Here's how the part is built. I have some questions about the finished solid (model axes, mm). Round coordinates to 2 decimals unless told otherwise and drop trailing zeros. Order: outer loops, then holes, each group sorted by start corner. A loop starts at its lowest first (then second) coordinate and runs counter-clockwise, first axis right, second up. Notation, with made-up numbers: (47, -4.75) -> (81, -4.75) arc R36 ccw to (81, 31.25) -> close; hole circle Ø8 at (87.25, 3). An arc over 180 degrees is marked (long way). Use a Markdown table: item, result. Add a question column.
(1) I want a section at D-D, the plane y = -31.5. Please give me the cut outline in (x, z).
(2) I want a section at C-C, the plane x = 13.5. Please give me the cut outline in (y, z).
(3) I want a section at B-B, the plane z = 0. Please give me the cut outline in (x, y).
(4) I want a section at A-A, the plane y = 66. Please give me the cut outline in (x, z).
(5) If I drill on probe 1 along X at (y, z) = (63.5, -5); probe 2 along Y at (x, z) = (1209, -74.5); probe 3 along X at (y, z) = (-22.5, 3.5), over which ranges is the centre line in solid material (lowest first)?
(6) I'm going to push flat-ended pins straight in: P1, Ø8, axis at y = 6, z = 33.5, coming from the +X side; P2, Ø5, axis at y = 93, z = -44.5, coming from the -X side; P3, Ø3, axis at y = -29.5, z = -15.5, coming from the +X side. Where does each tip first touch, or does it pass through?
from build123d import *

# Parameters (mm, degrees)
BOSS_EXTRUDE1_DEPTH = 100
SKETCH3_R           = 50
BOSS_EXTRUDE3_DEPTH = 50
SKETCH2_W           = 100
SKETCH2_H           = 100
CUT_EXTRUDE1_DEPTH  = 100
SKETCH4_W           = 200
SKETCH4_H           = 200
CUT_EXTRUDE2_DEPTH  = 10


with BuildPart() as part:
    # Sketch1 → Boss-Extrude1 (new body)
    with BuildSketch(Plane(origin=(0, 0, 0), x_dir=(1, 0, 0), z_dir=(0, 1, 0))):
        with BuildLine():
            Line((0, 150), (1150, 150))
            ThreePointArc((1150, 150), (1300, 0), (1150, -150))
            Line((1150, -150), (0, -150))
            ThreePointArc((0, -150), (-150, 0), (0, 150))
        make_face()
    extrude(amount=BOSS_EXTRUDE1_DEPTH)

    # Sketch3 → Boss-Extrude3 (add)
    with BuildSketch(Plane.XZ):
        with Locations(Location((0, 0, 0), (0, 0, 90))):
            Circle(SKETCH3_R)
    extrude(amount=BOSS_EXTRUDE3_DEPTH)

    # Sketch2 → Cut-Extrude1 (cut)
    with BuildSketch(Plane(origin=(0, 100, 0), x_dir=(1, 0, 0), z_dir=(0, 1, 0))):
        with Locations((1150, 0)):
            Rectangle(SKETCH2_W, SKETCH2_H)
    extrude(amount=-CUT_EXTRUDE1_DEPTH, mode=Mode.SUBTRACT)

    # Sketch4 → Cut-Extrude2 (cut)
    with BuildSketch(Plane(origin=(0, 100, 0), x_dir=(1, 0, 0), z_dir=(0, 1, 0))):
        with Locations((1150, 0)):
            Rectangle(SKETCH4_W, SKETCH4_H)
    extrude(amount=-CUT_EXTRUDE2_DEPTH, mode=Mode.SUBTRACT)


solid = part.part
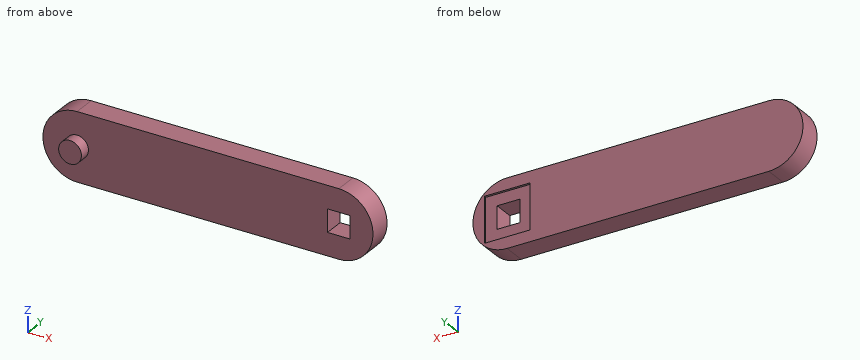
Taken from the geometry:
| question | item | result |
|---|---|---|
| 1 | outline | circle Ø100 at (0, 0) |
| 2 | outline | (-50, -48.14) -> (0, -48.14) -> (0, -150) -> (100, -150) -> (100, 150) -> (0, 150) -> (0, 48.14) -> (-50, 48.14) -> close |
| 3 | outline | (-150, 0) -> (-50, 0) -> (-50, -50) -> (50, -50) -> (50, 0) -> (1100, 0) -> (1100, 90) -> (1050, 90) -> (1050, 100) -> (-150, 100) -> close; (1200, 0) -> (1300, 0) -> (1300, 100) -> (1250, 100) -> (1250, 90) -> (1200, 90) -> close |
| 4 | outline | (0, -150) -> (1150, -150) arc R150 ccw to (1150, 150) -> (0, 150) arc R150 ccw to start; hole (1100, -50) -> (1200, -50) -> (1200, 50) -> (1100, 50) -> close |
| 5 | probe 1 | x = -149.92 to 1100, 1200 to 1299.92 |
| 5 | probe 2 | y = 0 to 90 |
| 5 | probe 3 | x = -49.88 to 49.88 |
| 6 | P1 | stops at x = 1297.07 |
| 6 | P2 | stops at x = -144 |
| 6 | P3 | stops at x = 48 |
